Job drawing, mm, ordinate dimensions from the low corner. One solid piece. Round coordinates to 2 decimals unless told otherwise and drop trailing zeros. Loops run counter-clockwise (first coordinate to the right, second up) from the corner with the lowest first, then second, coordinate; pieces in that order, holes last.
1) Band-saw the part on D-D, the plane y = 6. Write the cut outline in (x, z), then the cut area to 3 significant figures.
2) Band-saw the part on B-B, the plane z = 3.65. Write the cut outline in (x, y), then the cut area to 3 significant figures.
3) Drop flat-ended pins along their axis: P1, Ø1.5, axis at y = 46, z = 2, coming from the -X side; P2, Ø1.2, axis at y = 36.5, z = 3.5, coming from the -X side; P3, Ø2, axis at x = 3.5, z = 1, coming from the -Y side; P4, Ø1.2, axis at x = 1.5, z = 1, coming from the +Y side. Give the stop position or say it passes through.
4) Band-saw the part on A-A, the plane y = 41.5. Write the cut outline in (x, z).
5) Band-saw the part on C-C, the plane x = 34. Write the cut outline in (y, z).
6) Probe line 1 (X direction, y = 29.5, z = 4.25); line 2 (Y direction, x = 23, z = 3.4); line 3 (X direction, y = 37.5, z = 2.4). List the from-to ranges inside material, lowest first.
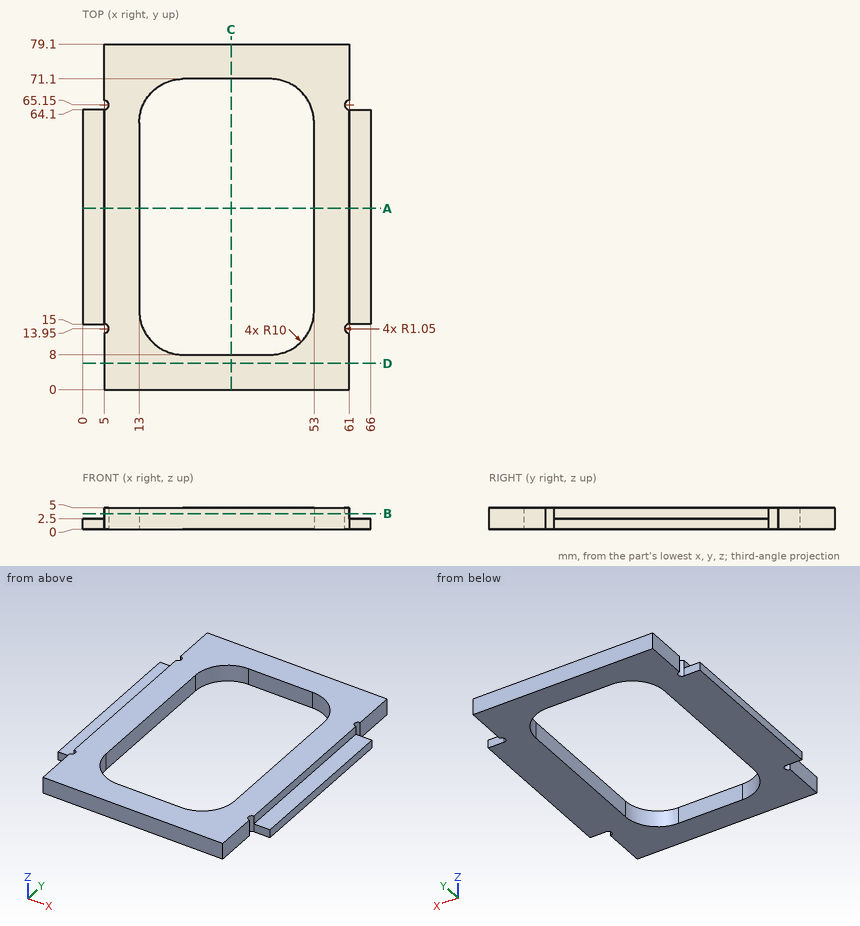
Reported:
1. outline: (5, 0) - (61, 0) - (61, 5) - (5, 5) - close
1. area: 280 mm2
2. outline: (5, 0) - (61, 0) - (61, 12.9) arc R1.05 cw to (61, 15) - (61, 64.1) arc R1.05 cw to (61, 66.2) - (61, 79.1) - (5, 79.1) - (5, 66.2) arc R1.05 cw to (5, 64.1) - (5, 15) arc R1.05 cw to (5, 12.9) - close; hole (13, 18) arc R10 ccw to (23, 8) - (43, 8) arc R10 ccw to (53, 18) - (53, 61.1) arc R10 ccw to (43, 71.1) - (23, 71.1) arc R10 ccw to (13, 61.1) - close
2. area: 1,980 mm2
3. P1: stops at x = 0
3. P2: stops at x = 5
3. P3: stops at y = 15
3. P4: stops at y = 64.1
4. outline: (0, 0) - (13, 0) - (13, 5) - (5, 5) - (5, 2.5) - (0, 2.5) - close; (53, 0) - (66, 0) - (66, 2.5) - (61, 2.5) - (61, 5) - (53, 5) - close
5. outline: (0, 0) - (8, 0) - (8, 5) - (0, 5) - close; (71.1, 0) - (79.1, 0) - (79.1, 5) - (71.1, 5) - close
6. line 1: x = 5 to 13, 53 to 61
6. line 2: y = 0 to 8, 71.1 to 79.1
6. line 3: x = 0 to 13, 53 to 66
